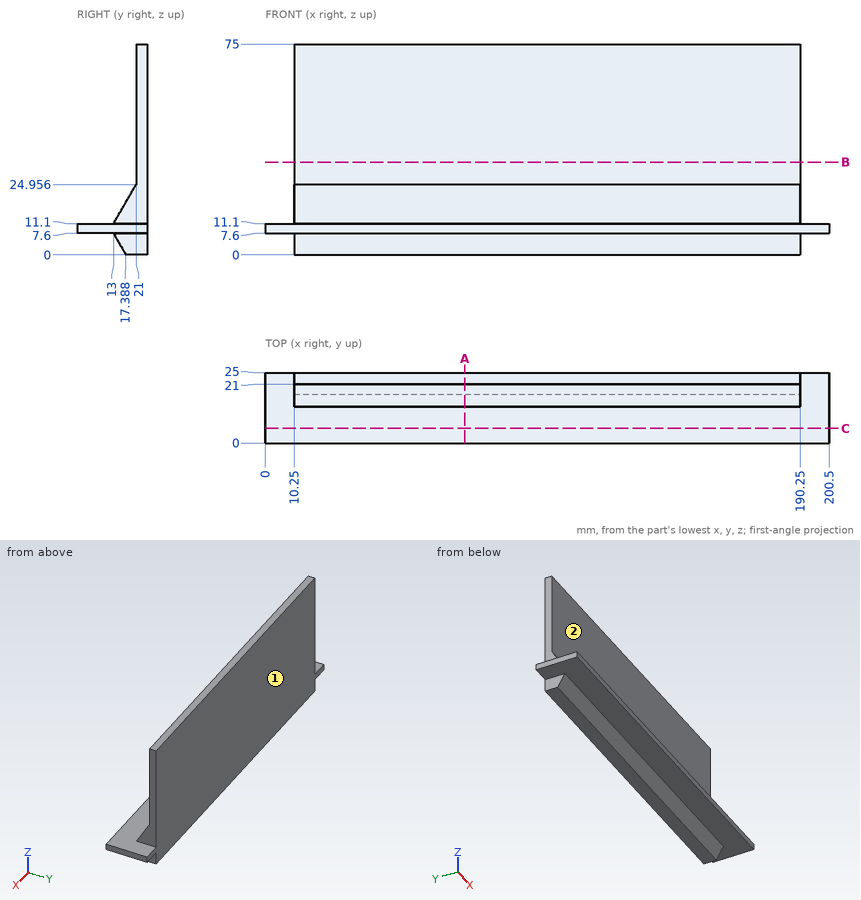
Check sheet for the drawn part. Datum: minimum x, y, z corner. Units: mm. A direction names the side the tool comes from. Coordinates: 2 decimals unless noted, no trailing zeros. Loops run counter-clockwise (first coordinate to the right, second up) from the corner with the lowest first, then second, coordinate; pieces in that order, holes last. Notation, with made-up numbers: (43, 66.25) -> (83, 66.25) arc R12 ccw to (83, 80.25) -> close; hole circle Ø1 at (-22.75, -26.5). An arc over 180 degrees is marked (long way). Answer as CSV lines item,"result".
1) Depth check by flat-ended pin: pin 1 (1 mm diameter, centred on x = 90.5, y = 12, fed in from +Z); pin 2 (13 mm diameter, centred on y = 17, z = 38.5, fed in from -X); pin 3 (6 mm diameter, centred on x = 129, z = 32, fed in from -Y); pin 4 (6 mm diameter, centred on y = 18.5, z = 5.5, fed in from -X). Enter the tip coordinate at first touch or a pass-through.
Found:
pin 1,"stops at z = 11.1"
pin 2,"stops at x = 10.25"
pin 3,"stops at y = 21"
pin 4,"stops at x = 0"
2) Cross-section at B-B, the plane z = 33. Record the cut outline in (x, y).
Found:
outline,"(10.25, 21) -> (190.25, 21) -> (190.25, 25) -> (10.25, 25) -> close"
3) Cross-section at A-A, the plane x = 71. Record the cut outline in (y, z), then the cut area to 3 significant figures.
Found:
outline,"(0, 7.6) -> (13, 7.6) -> (17.39, 0) -> (25, 0) -> (25, 75) -> (21, 75) -> (21, 24.96) -> (13, 11.1) -> (0, 11.1) -> close"
area,"473 mm2"
4) Cross-section at C-C, the plane y = 5.25. Record the cut outline in (x, z).
Found:
outline,"(0, 7.6) -> (200.5, 7.6) -> (200.5, 11.1) -> (0, 11.1) -> close"
5) Tool access check on the marked faces 1 and 2. Record the directions out of +Z, -Z, +X, -X, +Y, -Y that give a thin tool (end or side, any length) a straight path to the whole face; none if there is none.
Found:
face 1,"+Z, -Z, +X, -X, +Y"
face 2,"+Z, +X, -X, -Y"
6) Thickness scan on L1, parallel to Y at x = 99.5, z = 30.5; L2, parallel to Z at x = 132, y = 4.5; L3, parallel to X at y = 22.75, z = 59. Record the ranges inside material, lowest first. Write a range as from..to.
Found:
L1,"y = 21..25"
L2,"z = 7.6..11.1"
L3,"x = 10.25..190.25"
